from build123d import *

# Parameters (mm, degrees)
SKETCH1_R           = 6
SKETCH1_R_2         = 8.5
BOSS_EXTRUDE1_DEPTH = 8
FILLET1_R           = 5


with BuildPart() as part:
    # Sketch1 → Boss-Extrude1 (new body)
    with BuildSketch(Plane.XY):
        with BuildLine():
            ThreePointArc((12.5, -13.638181697), (0, 18.5), (-12.5, -13.638181697))
            Line((-12.5, -13.638181697), (-12.5, -23))
            ThreePointArc((-12.5, -23), (-6.5, -35), (-12.5, -47))
            Line((-12.5, -47), (-12.5, -152.456671403))
            Line((-12.5, -152.456671403), (0, -152.456671403))
            ThreePointArc((0, -152.456671403), (32.019441409, -179.184193262), (11.444366088, -215.464647068))
            ThreePointArc((11.444366088, -215.464647068), (-18.29086587, -232.773846738), (15.239317045, -240.488718511))
            ThreePointArc((15.239317045, -240.488718511), (57.52601951, -183.58870793), (12.5, -128.830749818))
            Line((12.5, -128.830749818), (12.5, -47))
            ThreePointArc((12.5, -47), (6.5, -35), (12.5, -23))
            Line((12.5, -23), (12.5, -13.638181697))
        make_face()
        with BuildLine():
            ThreePointArc((8.333859781, -228.327642037), (8.458362966, -229.159704854), (8.5, -230))
            ThreePointArc((8.5, -230), (-8.458362966, -230.840295146), (8.333859781, -228.327642037))
        make_face(mode=Mode.SUBTRACT)
        with Locations((0, -65)):
            Circle(SKETCH1_R, mode=Mode.SUBTRACT)
        Circle(SKETCH1_R_2, mode=Mode.SUBTRACT)
    extrude(amount=BOSS_EXTRUDE1_DEPTH)

    # Fillet1
    fillet1_edges = [part.edges().sort_by_distance(p)[0] for p in [
        (11.444366088, -215.464647068, 4),
        (-12.5, -152.456671403, 4),
        (-12.5, -13.638181697, 4),
        (12.5, -13.638181697, 4),
        (12.5, -128.830749818, 4),
        (15.239317045, -240.488718511, 4),
    ]]
    fillet(fillet1_edges, radius=FILLET1_R)


solid = part.part
CAD build for the part. Positions are in the model's coordinates, mm. A direction names the side the tool comes from. Give positions to 0.01 mm unless a question says otherwise; leave off trailing zeros. Loops run counter-clockwise (first coordinate to the right, second up) from the corner with the lowest first, then second, coordinate; pieces in that order, holes last. Notation, with made-up numbers: M 68,-13.75 L 98,-13.75 A13 cw 98,0.25 Z; hole C 66.5,27.25 d10. An arc over 180 degrees is marked long. Write each question's results on one line, items separated by ' | '.
Q1. Band-saw the part on B-B on y = -65. Write the cut outline in (x, z).
Geometry check:
outline: M -12.5,0 L -6,0 L -6,8 L -12.5,8 Z; M 6,0 L 12.5,0 L 12.5,8 L 6,8 Z
Q2. Flat gauge pins, fed straight in: P1, Ø15.5, axis at x = 0, y = -230, coming from the +Z side; P2, Ø1.5, axis at x = 36, z = 5, coming from the +Y side; P3, Ø3, axis at x = -7, y = -123, coming from the -Z side; P4, Ø4, axis at x = 25.5, z = 5.5, coming from the -Y side. Where does each tip first touch, or does it go through?
Geometry check:
P1: passes through | P2: stops at y = -139.52 | P3: stops at z = 0 | P4: stops at y = -237.53
Q3. Band-saw the part on D-D on y = -185.5. Write the cut outline in (x, z), and give its area (3 significant figures).
Geometry check:
outline: M 32.54,0 L 57.54,0 L 57.54,8 L 32.54,8 Z | area: 200 mm²
Q4. Mould opens along X. For faces 1 (the face through (11, -113, 8)), 2 (the face through (-1.301, -70.857, 3.944)), 3 (the face through (12.5, -19, 4)) say: pulls with the +X half, pulls with the -X half, needs draft (parallel to the pull), parting line crosses it, or undercut.
Geometry check:
face 1: needs draft | face 2: undercut | face 3: pulls with the +X half
Q5. Probe probe 1 along Y at (x, z) = (17, 7.25); probe 2 along X at (y, z) = (-120, 3); probe 3 along Y at (x, z) = (11, 6.75). List the from-to ranges inside material, lowest first.
Geometry check:
probe 1: y = -239.97 to -212.75, -157.25 to -130.03, -7.3 to 7.3 | probe 2: x = -12.5 to 12.5 | probe 3: y = -244.87 to -214.69, -154.37 to -45.71, -24.29 to 14.87
Q6. Which spindle directions (+Z, -Z, +X, -X, +Y, -Y) get a long thin tool onto all of the face, cutting with end or side? Do faces 4 (the face through (13.473, -127.919, 4.056)), 5 (the face through (-12.5, -97, 4)), 6 (the face through (4.57, 7.167, 3.944)). Say none if no direction does.
Geometry check:
face 4: +Z, -Z, +X | face 5: +Z, -Z, -X | face 6: +Z, -Z
Q7. Band-saw the part on A-A on y = 0. Write the cut outline in (x, z), and give its area (3 significant figures).
Geometry check:
outline: M -18.5,0 L -8.5,0 L -8.5,8 L -18.5,8 Z; M 8.5,0 L 18.5,0 L 18.5,8 L 8.5,8 Z | area: 160 mm²
Q8. Band-saw the part on C-C on z = 5.5. Give the number of separate pieces and of enclosed holes in the cut face, and give its area (3 significant figures).
Geometry check:
separate pieces: 1 | enclosed holes: 3 | area: 7,570 mm²
